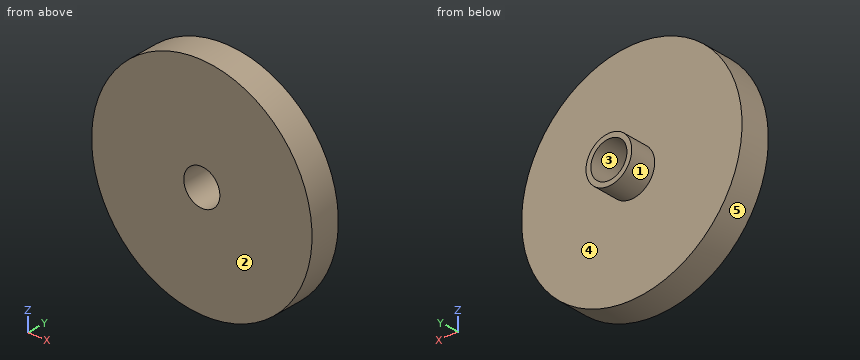
from build123d import *

# Parameters (mm, degrees)
SKETCH1_R           = 19.3929
BOSS_EXTRUDE1_DEPTH = 5.22
SKETCH2_R           = 3.175
CUT_EXTRUDE1_DEPTH  = 28.918050448
BOSS_EXTRUDE2_START = 4.5466
SKETCH3_R           = 4.0259
SKETCH3_R_2         = 3.175
BOSS_EXTRUDE2_DEPTH = 4.5466


with BuildPart() as part:
    # Sketch1 → Boss-Extrude1 (new body)
    with BuildSketch(Plane(origin=(0, 0, 0), x_dir=(1, 0, 0), z_dir=(0, 1, 0))):
        with Locations(Location((0, 0, 0), (0, 0, 270))):
            Circle(SKETCH1_R)
    extrude(amount=BOSS_EXTRUDE1_DEPTH)

    # Sketch2 → Cut-Extrude1 (cut, through all)
    with BuildSketch(Plane(origin=(0, 5.22, 0), x_dir=(1, 0, 0), z_dir=(0, 1, 0))):
        with Locations(Location((0, 0, 0), (0, 0, 270))):
            Circle(SKETCH2_R)
    extrude(amount=-CUT_EXTRUDE1_DEPTH, mode=Mode.SUBTRACT)

    # Sketch3 → Boss-Extrude2 (add)
    with BuildSketch(Plane(origin=(0, 5.22, 0), x_dir=(1, 0, 0), z_dir=(0, 1, 0)).offset(BOSS_EXTRUDE2_START)):
        with Locations(Location((0, 0, 0), (0, 0, 270))):
            Circle(SKETCH3_R)
        with Locations(Location((0, 0, 0), (0, 0, 270))):
            Circle(SKETCH3_R_2, mode=Mode.SUBTRACT)
    extrude(amount=-BOSS_EXTRUDE2_DEPTH)


solid = part.part
Input: part model. Units: mm. Frame: model coordinates. Face numbers are marked on the shaded views. A direction names the side the tool comes from. Round coordinates to 2 decimals unless told otherwise and drop trailing zeros. Write each loop counter-clockwise with the first axis right and the second up, starting at its lowest first coordinate (ties: lowest second). Pieces come first, ordered by that corner, then holes.
1) Reachability of the marked faces 1 and 2 from +Z, -Z, +X, -X, +Y, -Y: full face, straight path, thin tool, end or side. Return the list, or none.
2) Cut plane A-A (z = 0). Return the cut outline in (x, y) (3 decimals).
3) Draft query along Z for the marked faces 3, 4 and 5. Return one class per face: pulls with the +Z half, pulls with the -Z half, needs draft (parallel to the pull), parting line crosses it, or undercut.
4) Cut plane B-B (x = 0). Return the cut outline in (y, z) (3 decimals), then the cut area to 3 significant figures.
5) Contact query for flat-ended pins moving along their axis: P1, Ø4, axis at x = -5, y = 6.5, coming from the -Z side; P2, Ø5, axis at y = 2, z = -12, coming from the -X side; P3, Ø2, axis at y = 7.5, z = 3.5, coming from the +X side. Output: stop coordinate, or through.
6) Cut plane C-C (y = 2). Return the cut outline in (x, z) (3 decimals).
7) Ray query, L1, parallel to X at y = 6.25, z = 0 (3 decimals); L2, parallel to X at y = 4.5, z = 0 (3 decimals); L3, parallel to Y at x = -10, z = 14.5. Return the intervals inside material, ascending.
8) Cut plane D-D (z = 11.5). Return the cut outline in (x, y).
Geometry says:
1. face 1: +Y
1. face 2: +Z, -Z, +X, -X, -Y
2. outline: (-19.393, 0) - (-3.175, 0) - (-3.175, 9.767) - (-4.026, 9.767) - (-4.026, 5.22) - (-19.393, 5.22) - close; (3.175, 0) - (19.393, 0) - (19.393, 5.22) - (4.026, 5.22) - (4.026, 9.767) - (3.175, 9.767) - close
3. face 3: undercut
3. face 4: needs draft
3. face 5: parting line crosses it
4. outline: (0, -19.393) - (5.22, -19.393) - (5.22, -4.026) - (9.767, -4.026) - (9.767, -3.175) - (0, -3.175) - close; (0, 3.175) - (9.767, 3.175) - (9.767, 4.026) - (5.22, 4.026) - (5.22, 19.393) - (0, 19.393) - close
4. area: 177 mm2
5. P1: stops at z = -19.08
5. P2: stops at x = -16.91
5. P3: stops at x = 3.16
6. outline: circle Ø38.786 at (0, 0); hole circle Ø6.35 at (0, 0)
7. L1: x = -4.026 to -3.175, 3.175 to 4.026
7. L2: x = -19.393 to -3.175, 3.175 to 19.393
7. L3: y = 0 to 5.22
8. outline: (-15.62, 0) - (15.62, 0) - (15.62, 5.22) - (-15.62, 5.22) - close
